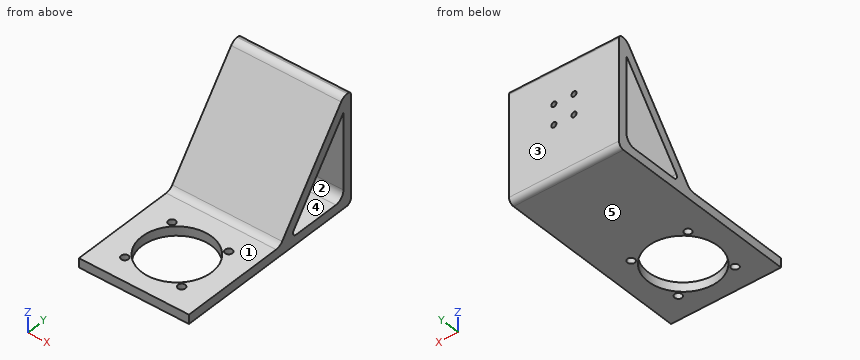
from build123d import *

# Parameters (mm, degrees)
BOSS_EXTRUDE1_DEPTH = 60
CUT_EXTRUDE2_REACH  = 108.6
SKETCH2_R           = 1.425
CUT_EXTRUDE3_REACH  = 62
SKETCH7_R           = 2
SKETCH7_R_2         = 19.05
FILLET2_R           = 5
FILLET4_R           = 5
FILLET5_R           = 2
FILLET6_R           = 2
FILLET7_R           = 3
FILLET8_R           = 5


with BuildPart() as part:
    # Sketch1 → Boss-Extrude1 (new body)
    with BuildSketch(Plane(origin=(0, 0, 0), x_dir=(0, 0, -1), z_dir=(1, 0, 0))):
        Polygon((-20.469264339, 47.094964584), (-20.469264339, 52.094964584), (39.530735661, 52.094964584), (39.530735661, -54.505035416), (34.530735661, -54.505035416), (34.530735661, 5.314612494), align=None)
        Polygon((-11.77256872, 47.094964584), (34.530735661, 11.920994403), (34.530735661, 47.094964584), align=None, mode=Mode.SUBTRACT)
    extrude(amount=-BOSS_EXTRUDE1_DEPTH)

    # Sketch2 → Cut-Extrude2 (cut, up to next)
    with BuildSketch(Plane(origin=(0, 52.094964584, 0), x_dir=(1, 0, 0), z_dir=(0, 1, 0)), mode=Mode.PRIVATE) as cut_extrude2_sk1:
        with Locations((-35.5, 10.030735661)):
            Circle(SKETCH2_R)
    cut_extrude2_tool1 = extrude(cut_extrude2_sk1.sketch, amount=-CUT_EXTRUDE2_REACH, mode=Mode.PRIVATE) & part.part
    add(cut_extrude2_tool1.solids().sort_by_distance((-35.5, 52.094965, -10.030736))[0], mode=Mode.SUBTRACT)
    # Sketch2 → Cut-Extrude2 (cut, up to next)
    with BuildSketch(Plane(origin=(0, 52.094964584, 0), x_dir=(1, 0, 0), z_dir=(0, 1, 0)), mode=Mode.PRIVATE) as cut_extrude2_sk2:
        with Locations((-24.5, 10.030735661)):
            Circle(SKETCH2_R)
    cut_extrude2_tool2 = extrude(cut_extrude2_sk2.sketch, amount=-CUT_EXTRUDE2_REACH, mode=Mode.PRIVATE) & part.part
    add(cut_extrude2_tool2.solids().sort_by_distance((-24.5, 52.094965, -10.030736))[0], mode=Mode.SUBTRACT)
    # Sketch2 → Cut-Extrude2 (cut, up to next)
    with BuildSketch(Plane(origin=(0, 52.094964584, 0), x_dir=(1, 0, 0), z_dir=(0, 1, 0)), mode=Mode.PRIVATE) as cut_extrude2_sk3:
        with Locations((-24.5, -0.969264339)):
            Circle(SKETCH2_R)
    cut_extrude2_tool3 = extrude(cut_extrude2_sk3.sketch, amount=-CUT_EXTRUDE2_REACH, mode=Mode.PRIVATE) & part.part
    add(cut_extrude2_tool3.solids().sort_by_distance((-24.5, 52.094965, 0.969264))[0], mode=Mode.SUBTRACT)
    # Sketch2 → Cut-Extrude2 (cut, up to next)
    with BuildSketch(Plane(origin=(0, 52.094964584, 0), x_dir=(1, 0, 0), z_dir=(0, 1, 0)), mode=Mode.PRIVATE) as cut_extrude2_sk4:
        with Locations((-35.5, -0.969264339)):
            Circle(SKETCH2_R)
    cut_extrude2_tool4 = extrude(cut_extrude2_sk4.sketch, amount=-CUT_EXTRUDE2_REACH, mode=Mode.PRIVATE) & part.part
    add(cut_extrude2_tool4.solids().sort_by_distance((-35.5, 52.094965, 0.969264))[0], mode=Mode.SUBTRACT)

    # Sketch7 → Cut-Extrude3 (cut, up to next)
    with BuildSketch(Plane(origin=(0, 0, -39.530735661), x_dir=(-1, 0, 0), z_dir=(0, 0, -1)), mode=Mode.PRIVATE) as cut_extrude3_sk1:
        with Locations((14.5, -10.805035416)):
            Circle(SKETCH7_R)
    cut_extrude3_tool1 = extrude(cut_extrude3_sk1.sketch, amount=-CUT_EXTRUDE3_REACH, mode=Mode.PRIVATE) & part.part
    add(cut_extrude3_tool1.solids().sort_by_distance((-14.5, -10.805035, -39.530736))[0], mode=Mode.SUBTRACT)
    # Sketch7 → Cut-Extrude3 (cut, up to next)
    with BuildSketch(Plane(origin=(0, 0, -39.530735661), x_dir=(-1, 0, 0), z_dir=(0, 0, -1)), mode=Mode.PRIVATE) as cut_extrude3_sk2:
        with Locations((45.5, -10.805035416)):
            Circle(SKETCH7_R)
    cut_extrude3_tool2 = extrude(cut_extrude3_sk2.sketch, amount=-CUT_EXTRUDE3_REACH, mode=Mode.PRIVATE) & part.part
    add(cut_extrude3_tool2.solids().sort_by_distance((-45.5, -10.805035, -39.530736))[0], mode=Mode.SUBTRACT)
    # Sketch7 → Cut-Extrude3 (cut, up to next)
    with BuildSketch(Plane(origin=(0, 0, -39.530735661), x_dir=(-1, 0, 0), z_dir=(0, 0, -1)), mode=Mode.PRIVATE) as cut_extrude3_sk3:
        with Locations((45.5, -41.805035416)):
            Circle(SKETCH7_R)
    cut_extrude3_tool3 = extrude(cut_extrude3_sk3.sketch, amount=-CUT_EXTRUDE3_REACH, mode=Mode.PRIVATE) & part.part
    add(cut_extrude3_tool3.solids().sort_by_distance((-45.5, -41.805035, -39.530736))[0], mode=Mode.SUBTRACT)
    # Sketch7 → Cut-Extrude3 (cut, up to next)
    with BuildSketch(Plane(origin=(0, 0, -39.530735661), x_dir=(-1, 0, 0), z_dir=(0, 0, -1)), mode=Mode.PRIVATE) as cut_extrude3_sk4:
        with Locations((14.5, -41.805035416)):
            Circle(SKETCH7_R)
    cut_extrude3_tool4 = extrude(cut_extrude3_sk4.sketch, amount=-CUT_EXTRUDE3_REACH, mode=Mode.PRIVATE) & part.part
    add(cut_extrude3_tool4.solids().sort_by_distance((-14.5, -41.805035, -39.530736))[0], mode=Mode.SUBTRACT)
    # Sketch7 → Cut-Extrude3 (cut, up to next)
    with BuildSketch(Plane(origin=(0, 0, -39.530735661), x_dir=(-1, 0, 0), z_dir=(0, 0, -1)), mode=Mode.PRIVATE) as cut_extrude3_sk5:
        with Locations((30, -26.305035416)):
            Circle(SKETCH7_R_2)
    cut_extrude3_tool5 = extrude(cut_extrude3_sk5.sketch, amount=-CUT_EXTRUDE3_REACH, mode=Mode.PRIVATE) & part.part
    add(cut_extrude3_tool5.solids().sort_by_distance((-30, -26.305035, -39.530736))[0], mode=Mode.SUBTRACT)

    # Fillet2
    fillet2_edges = [part.edges().sort_by_distance(p)[0] for p in [
        (-30, 47.094964584, -34.530735661),
    ]]
    fillet(fillet2_edges, radius=FILLET2_R)

    # Fillet4
    fillet4_edges = [part.edges().sort_by_distance(p)[0] for p in [
        (-30, 47.094964584, 20.469264339),
    ]]
    fillet(fillet4_edges, radius=FILLET4_R)

    # Fillet5
    fillet5_edges = [part.edges().sort_by_distance(p)[0] for p in [
        (-30, 11.920994403, -34.530735661),
    ]]
    fillet(fillet5_edges, radius=FILLET5_R)

    # Fillet6
    fillet6_edges = [part.edges().sort_by_distance(p)[0] for p in [
        (-30, 52.094964584, 20.469264339),
    ]]
    fillet(fillet6_edges, radius=FILLET6_R)

    # Fillet7
    fillet7_edges = [part.edges().sort_by_distance(p)[0] for p in [
        (-30, 52.094964584, -39.530735661),
    ]]
    fillet(fillet7_edges, radius=FILLET7_R)

    # Fillet8
    fillet8_edges = [part.edges().sort_by_distance(p)[0] for p in [
        (-30, 5.314612494, -34.530735661),
    ]]
    fillet(fillet8_edges, radius=FILLET8_R)


solid = part.part
Here's how the part is built. I have some questions about the finished solid (model axes, mm). Face numbers are marked on the shaded views. A direction names the side the tool comes from. Coordinates: 2 decimals unless noted, no trailing zeros. Write each loop counter-clockwise with the first axis right and the second up, starting at its lowest first coordinate (ties: lowest second). Pieces come first, ordered by that corner, then holes.
Item 1: I want a section at A-A on x = -30. Write out the boundary of the cut face in (y, z), and give its area (3 significant figures).
Item 2: On a 3-axis mill with a long thin cutter (end or side, diameter ignored), from which of +Z, -Z, +X, -X, +Y, -Y can I reach the whole of each face in a straight line? I mean the marked faces 4 and 5. Say none if no direction works.
Item 3: Will these pins go through, and if not, where does the flat tip stop? pin 1 (2.5 mm diameter, centred on x = -35.5, z = -10.03, fed in from +Y); pin 2 (17 mm diameter, centred on x = -34.5, y = -37.5, fed in from +Z); pin 3 (1 mm diameter, centred on x = -49.5, z = 10, fed in from -Y).
Item 4: If we mould it in two halves opening along Z, with no side actions, what happens to the marked faces 1, 2 and 3? For each: +Z half, -Z half, draft (parallel to the pull), parting line (faces both ways), or undercut.
Item 5: I want a section at B-B on x = -53.5. Write out the boundary of the cut face in (y, z).
Item 6: I want a section at C-C on y = -17. Write out the boundary of the cut face in (x, z).
Item 7: If I drill on line 1 (Z direction, x = -35.5, y = 50.15); line 2 (Z direction, x = -24.5, y = 49.55); line 3 (Y direction, x = -44.5, z = -27), over which ranges is the centre line in solid material (lowest first)?
Item 8: I want a section at D-D on z = -18. Write out the boundary of the cut face in (x, y).
Findings below:
1. outline: (-54.51, -39.53) - (-45.36, -39.53) - (-45.36, -34.53) - (-54.51, -34.53) - close; (-7.26, -39.53) - (49.09, -39.53) arc R3 ccw to (52.09, -36.53) - (52.09, 18.47) arc R2 ccw to (50.09, 20.47) - (49.58, 20.47) arc R5 ccw to (45.59, 18.49) - (6.82, -32.56) arc R5 cw to (2.83, -34.53) - (-7.26, -34.53) - close; hole (14.36, -31.32) arc R2 ccw to (15.95, -34.53) - (42.09, -34.53) arc R5 ccw to (47.09, -29.53) - (47.09, 11.77) - close
1. area: 958 mm2
2. face 4: +X, -X
2. face 5: -Z, +X, -X, +Y, -Y
3. pin 1: stops at y = 31.48
3. pin 2: stops at z = -34.53
3. pin 3: stops at y = 38.76
4. face 1: +Z half
4. face 2: undercut
4. face 3: draft
5. outline: (-54.51, -39.53) - (49.09, -39.53) arc R3 ccw to (52.09, -36.53) - (52.09, 18.47) arc R2 ccw to (50.09, 20.47) - (49.58, 20.47) arc R5 ccw to (45.59, 18.49) - (6.82, -32.56) arc R5 cw to (2.83, -34.53) - (-54.51, -34.53) - close; hole (14.36, -31.32) arc R2 ccw to (15.95, -34.53) - (42.09, -34.53) arc R5 ccw to (47.09, -29.53) - (47.09, 11.77) - close
6. outline: (-60, -39.53) - (-46.62, -39.53) - (-46.62, -34.53) - (-60, -34.53) - close; (-13.38, -39.53) - (0, -39.53) - (0, -34.53) - (-13.38, -34.53) - close
7. line 1: z = -39.34 to -11.46, -8.61 to -0.46, 2.39 to 20.47
7. line 2: z = -39.5 to -11.46, -8.61 to -0.46, 2.39 to 20.47
7. line 3: y = 11.04 to 17.64, 47.09 to 52.09
8. outline: (-60, 17.87) - (0, 17.87) - (0, 24.48) - (-60, 24.48) - close; (-60, 47.09) - (0, 47.09) - (0, 52.09) - (-60, 52.09) - close
